Build history of the part. All positions in model axes, mm. Give positions to 0.01 mm unless a question says otherwise; leave off trailing zeros. Order: outer loops, then holes, each group sorted by start corner. A loop starts at its lowest first (then second) coordinate and runs counter-clockwise, first axis right, second up. Notation, with made-up numbers: M 77,36.5 L 95,36.5 A25 ccw 95,67.5 Z; hole C 28.5,-27 d2. An arc over 180 degrees is marked long. One line per item, written item: value. Start each with the question number.
from build123d import *

# Parameters (mm, degrees)
SKETCH1_R           = 3.25
BOSS_EXTRUDE1_DEPTH = 5
CUT_EXTRUDE1_START  = -6
SKETCH2_R           = 2.075
CUT_EXTRUDE1_DEPTH  = 7
FILLET1_R           = 4


with BuildPart() as part:
    # Sketch1 → Boss-Extrude1 (new body)
    with BuildSketch(Plane(origin=(0, 0, 0), x_dir=(1, 0, 0), z_dir=(0, 1, 0))):
        Polygon((-59.15, -15), (-82.443714059, -101.933324366), (-63.125197533, -107.109705268), (-39.831483474, -20.176380902), (-39.15, -17.633049952), (-39.15, -15), (-39.15, 15), (-59.15, 15), align=None)
        with Locations((-49.15, 0)):
            Circle(SKETCH1_R, mode=Mode.SUBTRACT)
    extrude(amount=BOSS_EXTRUDE1_DEPTH)

    # Sketch2 → Cut-Extrude1 (cut)
    with BuildSketch(Plane(origin=(0, 5, 0), x_dir=(1, 0, 0), z_dir=(0, 1, 0)).offset(CUT_EXTRUDE1_START)):
        with Locations((-49.15, 8)):
            Circle(SKETCH2_R)
    cut_extrude1 = extrude(amount=CUT_EXTRUDE1_DEPTH, mode=Mode.SUBTRACT)

    # Mirror1: Cut-Extrude1 across plane
    add(cut_extrude1.mirror(Plane.XY), mode=Mode.SUBTRACT)

    # Fillet1
    fillet1_edges = [part.edges().sort_by_distance(p)[0] for p in [
        (-39.15, 2.5, 17.633049952),
        (-63.125197533, 2.5, 107.109705268),
        (-82.443714059, 2.5, 101.933324366),
        (-59.15, 2.5, 15),
        (-59.15, 2.5, -15),
        (-39.15, 2.5, -15),
    ]]
    fillet(fillet1_edges, radius=FILLET1_R)


solid = part.part
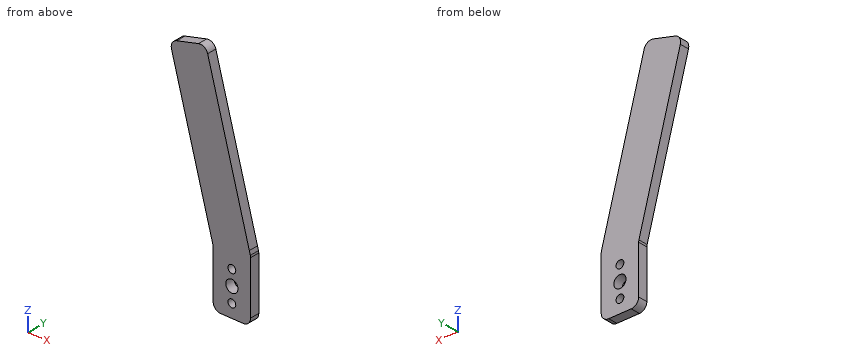
1) Slice it at A-A (z = -8). List the corners of the cut face in (x, y) (3 decimals).
2) Slice it at C-C (x = -49.15). List the corners of the cut face in (y, z) (3 decimals), plus the area to 3 significant figures.
3) Drop a flat-ended pin along its axis: P1, Ø1.5, axis at y = 1.5, z = -2, coming from the -X side. Give the stop position or say it passes through.
4) Slice it at B-B (y = 3.4). List the corners of the cut face in (x, z) (3 decimals), plus the area to 3 significant figures.
5) Drill centre lines: line 1 (X direction, y = 2.4, z = 0); line 2 (X direction, y = 2.25, z = 13.5); line 3 (X direction, y = 2, z = 19.5). Where is each one in solid material? Low to high.
6) Slice it at D-D (x = -69.5). List the corners of the cut face in (y, z), plus the area to 3 significant figures.
Results list:
1. outline: M -59.15,0 L -51.225,0 L -51.225,5 L -59.15,5 Z; M -47.075,0 L -39.15,0 L -39.15,5 L -47.075,5 Z
2. outline: M 0,-15 L 5,-15 L 5,-10.075 L 0,-10.075 Z; M 0,-5.925 L 5,-5.925 L 5,-3.25 L 0,-3.25 Z; M 0,3.25 L 5,3.25 L 5,5.925 L 0,5.925 Z; M 0,10.075 L 5,10.075 L 5,54.954 L 0,54.954 Z
2. area: 276 mm²
3. P1: stops at x = -59.15
4. outline: M -81.408,98.07 L -59.286,15.509 A4 cw -59.15,14.473 L -59.15,-11 A4 ccw -55.15,-15 L -43.15,-15 A4 ccw -39.15,-11 L -39.15,17.106 A4 ccw -39.286,18.142 L -62.09,103.246 A4 ccw -66.989,106.074 L -78.58,102.969 A4 ccw Z; hole C -49.15,0 d6.5; hole C -49.15,-8 d4.15; hole C -49.15,8 d4.15
4. area: 2,380 mm²
5. line 1: x = -59.15 to -52.4, -45.9 to -39.15
5. line 2: x = -59.15 to -39.15
5. line 3: x = -60.36 to -39.65
6. outline: M 0,53.63 L 5,53.63 L 5,105.4 L 0,105.4 Z
6. area: 259 mm²
